The model under review builds one solid part; all positions refer to its coordinate system, in mm. Coordinates: 2 decimals unless noted, no trailing zeros. Loops run counter-clockwise (first coordinate to the right, second up) from the corner with the lowest first, then second, coordinate; pieces in that order, holes last. Notation, with made-up numbers: M 54.25,68 L 83.25,68 A19 ccw 83.25,76 Z; hole C -12.5,53 d6. An arc over 180 degrees is marked long. One line per item, written item: value.
```python
from build123d import *

# Parameters (mm, degrees)
F1_DEPTH = 2.5


with BuildPart() as f1:
    # F0 (on Front) → F1 (new body, symmetric)
    with BuildSketch(Plane.XZ):
        with BuildLine():
            Line((31, 0), (40, 0))
            ThreePointArc((40, 0), (39.921490373, 2.5049164455), (39.68626968, 4.9999998882))
            Line((39.68626968, 4.9999998882), (30.5941170998, 4.9999998882))
            ThreePointArc((30.5941170998, 4.9999998882), (30.8983626596, 2.5082234655), (31, 0))
        make_face()
        with BuildLine():
            ThreePointArc((39.686269666, -5), (39.9214903695, -2.5049165017), (40, 0))
            Line((40, 0), (31, 0))
            ThreePointArc((31, 0), (30.8983626551, -2.5082235219), (30.5941170816, -5))
            Line((30.5941170816, -5), (39.686269666, -5))
        make_face()
        with BuildLine():
            Line((30.5941170998, 4.9999998882), (39.68626968, 4.9999998882))
            ThreePointArc((39.68626968, 4.9999998882), (28.2842712674, 28.2842712275), (4.9999999441, 39.686269673))
            Line((4.9999998882, 39.686269673), (4.9999998882, 30.5941170907))
            ThreePointArc((4.9999999441, 30.5941170907), (21.9203102368, 21.9203101968), (30.5941170998, 4.9999998882))
        make_face()
        with BuildLine():
            ThreePointArc((4.9999998882, -39.68626968), (28.2842712076, -28.2842712873), (39.686269666, -5))
            Line((39.686269666, -5), (30.5941170816, -5))
            ThreePointArc((30.5941170816, -5), (21.9203101767, -21.9203102568), (4.9999998882, -30.5941170998))
            Line((4.9999998882, -30.5941170998), (4.9999998882, -39.68626968))
        make_face()
        with BuildLine():
            Line((4.9999998882, 30.5941170907), (4.9999998882, 39.686269673))
            ThreePointArc((4.9999999441, 39.686269673), (2.5049164736, 39.9214903712), (0, 40))
            Line((0, 40), (0, 31))
            ThreePointArc((0, 31), (2.5082234937, 30.8983626574), (4.9999999441, 30.5941170907))
        make_face()
        with BuildLine():
            ThreePointArc((0, -40), (2.5049164455, -39.921490373), (4.9999998882, -39.68626968))
            Line((4.9999998882, -39.68626968), (4.9999998882, -30.5941170998))
            ThreePointArc((4.9999998882, -30.5941170998), (2.5082234655, -30.8983626596), (0, -31))
            Line((0, -31), (0, -40))
        make_face()
        with BuildLine():
            Line((0, 31), (0, 40))
            ThreePointArc((0, 40), (-2.5049164455, 39.921490373), (-4.9999998882, 39.68626968))
            Line((-4.9999998882, 39.68626968), (-4.9999998882, 30.5941170998))
            ThreePointArc((-4.9999998882, 30.5941170998), (-2.5082234655, 30.8983626596), (0, 31))
        make_face()
        with BuildLine():
            ThreePointArc((-5, -39.686269666), (-2.5049165017, -39.9214903695), (0, -40))
            Line((0, -40), (0, -31))
            ThreePointArc((0, -31), (-2.5082235219, -30.8983626551), (-5, -30.5941170816))
            Line((-5, -30.5941170816), (-5, -39.686269666))
        make_face()
        with BuildLine():
            Line((-4.9999998882, 30.5941170998), (-4.9999998882, 39.68626968))
            ThreePointArc((-4.9999998882, 39.68626968), (-28.2842712076, 28.2842712873), (-39.686269666, 5))
            Line((-39.686269666, 5), (-30.5941170816, 5))
            ThreePointArc((-30.5941170816, 5), (-21.9203101767, 21.9203102568), (-4.9999998882, 30.5941170998))
        make_face()
        with BuildLine():
            ThreePointArc((-39.68626968, -4.9999998882), (-28.2842712873, -28.2842712076), (-5, -39.686269666))
            Line((-5, -39.686269666), (-5, -30.5941170816))
            ThreePointArc((-5, -30.5941170816), (-21.9203102568, -21.9203101767), (-30.5941170998, -4.9999998882))
            Line((-30.5941170998, -4.9999998882), (-39.68626968, -4.9999998882))
        make_face()
        with BuildLine():
            Line((-30.5941170816, 5), (-39.686269666, 5))
            ThreePointArc((-39.686269666, 5), (-39.9214903695, 2.5049165017), (-40, 0))
            Line((-40, 0), (-31, 0))
            ThreePointArc((-31, 0), (-30.8983626551, 2.5082235219), (-30.5941170816, 5))
        make_face()
        with BuildLine():
            ThreePointArc((-40, 0), (-39.921490373, -2.5049164455), (-39.68626968, -4.9999998882))
            Line((-39.68626968, -4.9999998882), (-30.5941170998, -4.9999998882))
            ThreePointArc((-30.5941170998, -4.9999998882), (-30.8983626596, -2.5082234655), (-31, 0))
            Line((-31, 0), (-40, 0))
        make_face()
        with BuildLine():
            Line((4.9999998882, 5.5901699937), (4.9999998882, 30.5941170907))
            ThreePointArc((4.9999999441, 30.5941170907), (2.5082234937, 30.8983626574), (0, 31))
            Line((0, 31), (0, 7.5))
            ThreePointArc((0, 7.5), (2.6761656383, 7.0062927056), (4.9999999441, 5.5901699937))
        make_face()
        with BuildLine():
            Line((0, 7.5), (0, 31))
            ThreePointArc((0, 31), (-2.5082234655, 30.8983626596), (-4.9999998882, 30.5941170998))
            Line((-4.9999998882, 30.5941170998), (-4.9999998882, 5.5901700437))
            ThreePointArc((-4.9999998882, 5.5901700437), (-2.6761656033, 7.006292719), (0, 7.5))
        make_face()
        with BuildLine():
            Line((-5.5901699437, 5), (-30.5941170816, 5))
            ThreePointArc((-30.5941170816, 5), (-30.8983626551, 2.5082235219), (-31, 0))
            Line((-31, 0), (-7.5, 0))
            ThreePointArc((-7.5, 0), (-7.0062926922, 2.6761656733), (-5.5901699437, 5))
        make_face()
        with BuildLine():
            ThreePointArc((-31, 0), (-30.8983626596, -2.5082234655), (-30.5941170998, -4.9999998882))
            Line((-30.5941170998, -4.9999998882), (-5.5901700437, -4.9999998882))
            ThreePointArc((-5.5901700437, -4.9999998882), (-7.006292719, -2.6761656033), (-7.5, 0))
            Line((-7.5, 0), (-31, 0))
        make_face()
        with BuildLine():
            ThreePointArc((-5, -30.5941170816), (-2.5082235219, -30.8983626551), (0, -31))
            Line((0, -31), (0, -7.5))
            ThreePointArc((0, -7.5), (-2.6761656733, -7.0062926922), (-5, -5.5901699437))
            Line((-5, -5.5901699437), (-5, -30.5941170816))
        make_face()
        with BuildLine():
            ThreePointArc((0, -31), (2.5082234655, -30.8983626596), (4.9999998882, -30.5941170998))
            Line((4.9999998882, -30.5941170998), (4.9999998882, -5.5901700437))
            ThreePointArc((4.9999998882, -5.5901700437), (2.6761656033, -7.006292719), (0, -7.5))
            Line((0, -7.5), (0, -31))
        make_face()
        with BuildLine():
            ThreePointArc((30.5941170816, -5), (30.8983626551, -2.5082235219), (31, 0))
            Line((31, 0), (7.5, 0))
            ThreePointArc((7.5, 0), (7.0062926922, -2.6761656733), (5.5901699437, -5))
            Line((5.5901699437, -5), (30.5941170816, -5))
        make_face()
        with BuildLine():
            Line((7.5, 0), (31, 0))
            ThreePointArc((31, 0), (30.8983626596, 2.5082234655), (30.5941170998, 4.9999998882))
            Line((30.5941170998, 4.9999998882), (5.5901700437, 4.9999998882))
            ThreePointArc((5.5901700437, 4.9999998882), (7.006292719, 2.6761656033), (7.5, 0))
        make_face()
        with BuildLine():
            Line((4.9999999255, 0), (7.5, 0))
            ThreePointArc((7.5, 0), (7.006292719, 2.6761656033), (5.5901700437, 4.9999998882))
            Line((5.5901700437, 4.9999998882), (4.9999999441, 4.9999998882))
            Line((4.9999998882, 4.9999998882), (4.9999998882, 0))
        make_face()
        with BuildLine():
            Line((2.5, 0), (4.9999999255, 0))
            Line((4.9999998882, 0), (4.9999998882, 4.9999998882))
            Line((4.9999999441, 4.9999998882), (0, 4.9999998882))
            Line((0, 4.9999999441), (0, 2.5))
            ThreePointArc((0, 2.5), (1.767766953, 1.767766953), (2.5, 0))
        make_face()
        with BuildLine():
            Line((4.9999998882, 4.9999998882), (4.9999998882, 5.5901699937))
            ThreePointArc((4.9999999441, 5.5901699937), (2.6761656383, 7.0062927056), (0, 7.5))
            Line((0, 7.5), (0, 4.9999999441))
            Line((0, 4.9999998882), (4.9999999441, 4.9999998882))
        make_face()
        with BuildLine():
            Line((0, 4.9999999441), (0, 7.5))
            ThreePointArc((0, 7.5), (-2.6761656033, 7.006292719), (-4.9999998882, 5.5901700437))
            Line((-4.9999998882, 5.5901700437), (-4.9999998882, 5))
            Line((-4.9999998882, 5), (0, 5))
        make_face()
        with BuildLine():
            Line((0, 2.5), (0, 4.9999999441))
            Line((0, 5), (-4.9999998882, 5))
            Line((-4.9999998882, 5), (-4.9999998882, 0))
            Line((-4.9999999441, 0), (-2.5, 0))
            ThreePointArc((-2.5, 0), (-1.767766953, 1.767766953), (0, 2.5))
        make_face()
        with BuildLine():
            Line((-4.9999998882, 0), (-4.9999998882, 5))
            Line((-4.9999998882, 5), (-5.5901699437, 5))
            ThreePointArc((-5.5901699437, 5), (-7.0062926922, 2.6761656733), (-7.5, 0))
            Line((-7.5, 0), (-4.9999999441, 0))
        make_face()
        with BuildLine():
            Line((-5.5901700437, -4.9999998882), (-5, -4.9999998882))
            Line((-5, -4.9999998882), (-5, 0))
            Line((-4.9999999441, 0), (-7.5, 0))
            ThreePointArc((-7.5, 0), (-7.006292719, -2.6761656033), (-5.5901700437, -4.9999998882))
        make_face()
        with BuildLine():
            Line((-5, -4.9999998882), (0, -4.9999998882))
            Line((0, -4.9999999441), (0, -2.5))
            ThreePointArc((0, -2.5), (-1.767766953, -1.767766953), (-2.5, 0))
            Line((-2.5, 0), (-4.9999999441, 0))
            Line((-5, 0), (-5, -4.9999998882))
        make_face()
        with BuildLine():
            Line((4.9999998882, -5), (4.9999998882, 0))
            Line((4.9999999255, 0), (2.5, 0))
            ThreePointArc((2.5, 0), (1.767766953, -1.767766953), (0, -2.5))
            Line((0, -2.5), (0, -4.9999999441))
            Line((0, -5), (4.9999998882, -5))
        make_face()
        with BuildLine():
            ThreePointArc((5.5901699437, -5), (7.0062926922, -2.6761656733), (7.5, 0))
            Line((7.5, 0), (4.9999999255, 0))
            Line((4.9999998882, 0), (4.9999998882, -5))
            Line((4.9999998882, -5), (5.5901699437, -5))
        make_face()
        with BuildLine():
            ThreePointArc((0, -7.5), (2.6761656033, -7.006292719), (4.9999998882, -5.5901700437))
            Line((4.9999998882, -5.5901700437), (4.9999998882, -5))
            Line((4.9999998882, -5), (0, -5))
            Line((0, -4.9999999441), (0, -7.5))
        make_face()
        with BuildLine():
            Line((-4.9999998882, 5), (-4.9999998882, 5.5901700437))
            ThreePointArc((-4.9999998882, 5.5901700437), (-5.3033008059, 5.3033009119), (-5.5901699437, 5))
            Line((-5.5901699437, 5), (-4.9999998882, 5))
        make_face()
        with BuildLine():
            ThreePointArc((-5.5901700437, -4.9999998882), (-5.3033009119, -5.3033008059), (-5, -5.5901699437))
            Line((-5, -5.5901699437), (-5, -4.9999998882))
            Line((-5, -4.9999998882), (-5.5901700437, -4.9999998882))
        make_face()
        with BuildLine():
            ThreePointArc((-5, -5.5901699437), (-2.6761656733, -7.0062926922), (0, -7.5))
            Line((0, -7.5), (0, -4.9999999441))
            Line((0, -4.9999998882), (-5, -4.9999998882))
            Line((-5, -4.9999998882), (-5, -5.5901699437))
        make_face()
        with BuildLine():
            ThreePointArc((4.9999998882, -5.5901700437), (5.3033008059, -5.3033009119), (5.5901699437, -5))
            Line((5.5901699437, -5), (4.9999998882, -5))
            Line((4.9999998882, -5), (4.9999998882, -5.5901700437))
        make_face()
        with BuildLine():
            Line((4.9999999441, 4.9999998882), (5.5901700437, 4.9999998882))
            ThreePointArc((5.5901700437, 4.9999998882), (5.3033008854, 5.3033008324), (4.9999999441, 5.5901699937))
            Line((4.9999998882, 5.5901699937), (4.9999998882, 4.9999998882))
        make_face()
    extrude(amount=F1_DEPTH, both=True)


solid = f1.part
```
(1) Add section B-B on y = -1.35. State the section outline as (x, z) points, then the cut area to 3 significant figures.
Checks:
outline: C 0,0 d80; hole M -30.59,-5 A31 ccw -5,-30.59 L -5,-5.59 A7.5 cw -5.59,-5 Z; hole M -30.59,5 L -5.59,5 A7.5 cw -5,5.59 L -5,30.59 A31 ccw Z; hole C 0,0 d5; hole M 5,-30.59 A31 ccw 30.59,-5 L 5.59,-5 A7.5 cw 5,-5.59 Z; hole M 5,5.59 A7.5 cw 5.59,5 L 30.59,5 A31 ccw 5,30.59 Z
area: 3,120 mm^2
(2) Add section C-C on z = -20.5. State the section outline as (x, y) points, then the cut area to 3 significant figures.
Checks:
outline: M -34.35,-2.5 L -23.25,-2.5 L -23.25,2.5 L -34.35,2.5 Z; M -5,-2.5 L 5,-2.5 L 5,2.5 L -5,2.5 Z; M 23.25,-2.5 L 34.35,-2.5 L 34.35,2.5 L 23.25,2.5 Z
area: 161 mm^2
(3) Add section D-D on x = 34. State the section outline as (y, z) points, then the cut area to 3 significant figures.
Checks:
outline: M -2.5,-21.07 L 2.5,-21.07 L 2.5,21.07 L -2.5,21.07 Z
area: 211 mm^2
(4) Add section A-A on x = -18.5. State the section outline as (y, z) points, then the cut area to 3 significant figures.
Checks:
outline: M -2.5,-35.46 L 2.5,-35.46 L 2.5,-24.87 L -2.5,-24.87 Z; M -2.5,-5 L 2.5,-5 L 2.5,5 L -2.5,5 Z; M -2.5,24.87 L 2.5,24.87 L 2.5,35.46 L -2.5,35.46 Z
area: 156 mm^2
(5) To check wall thickness, follow L1, parallel to Z at x = -8, y = 1.25; L2, parallel to Z at x = 26, y = 2.2; L3, parallel to X at y = 1.5, z = -24. State the ranges of each line that lie inside material, in increasing order. Write a range as [from, to].
Checks:
L1: [-39.19, -29.95], [-5, 5], [29.95, 39.19]
L2: [-30.4, -16.88], [-5, 5], [16.88, 30.4]
L3: [-32, -19.62], [-5, 5], [19.62, 32]
(6) Insertion check: pin 1 Ø0.8 at (y, z) = (1.5, -14) entering from +X; pin 2 Ø1.2 at (x, y) = (-18.5, -1.5) entering from +Z; pin 3 Ø0.8 at (y, z) = (-1.5, -17.5) entering from +X. Each pin has a flat end and moves straight along its axis. Give the tip position at first contact, or say it passes through.
Checks:
pin 1: x = 37.62
pin 2: z = 35.77
pin 3: x = 36.16
